For this review, take the finished solid that the model builds, in its own axes (mm). A direction names the side the tool comes from. Coordinates: 2 decimals unless noted, no trailing zeros. Write each loop counter-clockwise with the first axis right and the second up, starting at its lowest first coordinate (ties: lowest second). Pieces come first, ordered by that corner, then holes. Notation, with made-up numbers: (52.25, -0.5) - (61.25, -0.5) arc R27 ccw to (61.25, 30.5) - close; hole circle Ø5 at (11.5, -39.5). An arc over 180 degrees is marked (long way). Write each question's results on one line, items separated by ' | '.
from build123d import *

# Parameters (mm, degrees)
F0_W     = 4
F0_H     = 10
F0_W_2   = 9
F0_W_3   = 20.5
F1_DEPTH = 6.5
F2_DEPTH = 3.55
F3_DEPTH = 1.95
F4_R     = 3.5
F5_DEPTH = 25


with BuildPart() as f1:
    # F0 (on Top) → F1 (new body)
    with BuildSketch(Plane.XY):
        with Locations((-21.25, 5)):
            Rectangle(F0_W, F0_H)
        with Locations((-14.75, 5)):
            Rectangle(F0_W_2, F0_H)
        with Locations((0, 5)):
            Rectangle(F0_W_3, F0_H)
        with Locations((14.75, 5)):
            Rectangle(F0_W_2, F0_H)
        with Locations((21.25, 5)):
            Rectangle(F0_W, F0_H)
    extrude(amount=F1_DEPTH)

    # F0 (on Top) → F2 (cut)
    with BuildSketch(Plane.XY):
        with Locations((-14.75, 5)):
            Rectangle(F0_W_2, F0_H)
        with Locations((0, 5)):
            Rectangle(F0_W_3, F0_H)
        with Locations((14.75, 5)):
            Rectangle(F0_W_2, F0_H)
    extrude(amount=F2_DEPTH, mode=Mode.SUBTRACT)

    # F0 (on Top) → F3 (join)
    with BuildSketch(Plane.XY):
        with Locations((-14.75, 5)):
            Rectangle(F0_W_2, F0_H)
        with Locations((14.75, 5)):
            Rectangle(F0_W_2, F0_H)
    extrude(amount=F3_DEPTH)

    # F4 (on face) → F5 (join)
    with BuildSketch(Plane.XY.offset(6.5)):
        with BuildLine():
            ThreePointArc((0, 0), (3.535534, 1.464466), (5, 5))
            ThreePointArc((5, 5), (3.535534, 8.535534), (0, 10))
            ThreePointArc((0, 10), (-5, 5), (0, 0))
        make_face()
        with Locations((0, 5)):
            Circle(F4_R, mode=Mode.SUBTRACT)
    extrude(amount=F5_DEPTH)


solid = f1.part
Q1. Take a section at D-D on x = -2.5. State the section outline as (y, z) points.
Results found:
outline: (0, 3.55) - (10, 3.55) - (10, 6.5) - (9.33, 6.5) - (9.33, 31.5) - (7.45, 31.5) - (7.45, 6.5) - (2.55, 6.5) - (2.55, 31.5) - (0.67, 31.5) - (0.67, 6.5) - (0, 6.5) - close
Q2. Take a section at A-A on x = 17. State the section outline as (y, z) points.
Results found:
outline: (0, 0) - (10, 0) - (10, 1.95) - (0, 1.95) - close; (0, 3.55) - (10, 3.55) - (10, 6.5) - (0, 6.5) - close
Q3. Wall thickness on line 1 along Z through (x, y) = (-15, 6.75); line 2 along Y through (x, z) = (0, 19); line 3 along X through (y, z) = (3, 1): over which ranges is each line inside the solid? List them lowest first. Write a range as from..to.
Results found:
line 1: 0..1.95, 3.55..6.5 | line 2: 0..1.5, 8.5..10 | line 3: -23.25..-10.25, 10.25..23.25
Q4. Mouldability with a two-part tool opening along Y and no side actions: class faces 4 (the face through (1.615, 1.895, 18.825)), 5 (the face through (15, 5, 1.95)), 6 (the face through (0, 5, 6.5)), 7 (the face through (0, 0, 4)) as pulls with the +Y half, pulls with the -Y half, needs draft (parallel to the pull), parting line crosses it, or undercut.
Results found:
face 4: undercut | face 5: needs draft | face 6: undercut | face 7: pulls with the -Y half
Q5. For faces 1 (the face through (-17, 5, 0)), 2 (the face through (-19.25, 5, 3)), 3 (the face through (10.25, 5, 1)), list the 3-axis set-ups (+Z, -Z, +X, -X, +Y, -Y) from which the entire face can be reached by the end or side of a thin tool; tool diameter is ignored.
Results found:
face 1: -Z, +X, -X, +Y, -Y | face 2: +Y, -Y | face 3: -Z, +Y, -Y
Q6. Take a section at C-C on z = 18.5. State the section outline as (x, y) points.
Results found:
outline: circle Ø10 at (0, 5); hole circle Ø7 at (0, 5)
Q7. For pin 1 (5 mm diameter, centred on x = 6, y = 5, fed in from -Z); pin 2 (8 mm diameter, centred on x = 0.5, z = 23.5, fed in from -Y); pin 3 (2 mm diameter, centred on y = 1.5, z = 19, fed in from +X); pin 4 (4 mm diameter, centred on y = 4.5, z = 9.5, fed in from -X), all flat-tipped, find the tip position at first contact; note any pin that passes through.
Results found:
pin 1: z = 3.55 | pin 2: y = 0 | pin 3: x = 4.33 | pin 4: x = -5
Q8. Take a section at B-B on y = 1. State the section outline as (x, z) points.
Results found:
outline: (-23.25, 0) - (-10.25, 0) - (-10.25, 1.95) - (-19.25, 1.95) - (-19.25, 3.55) - (19.25, 3.55) - (19.25, 1.95) - (10.25, 1.95) - (10.25, 0) - (23.25, 0) - (23.25, 6.5) - (3, 6.5) - (3, 31.5) - (-3, 31.5) - (-3, 6.5) - (-23.25, 6.5) - close
